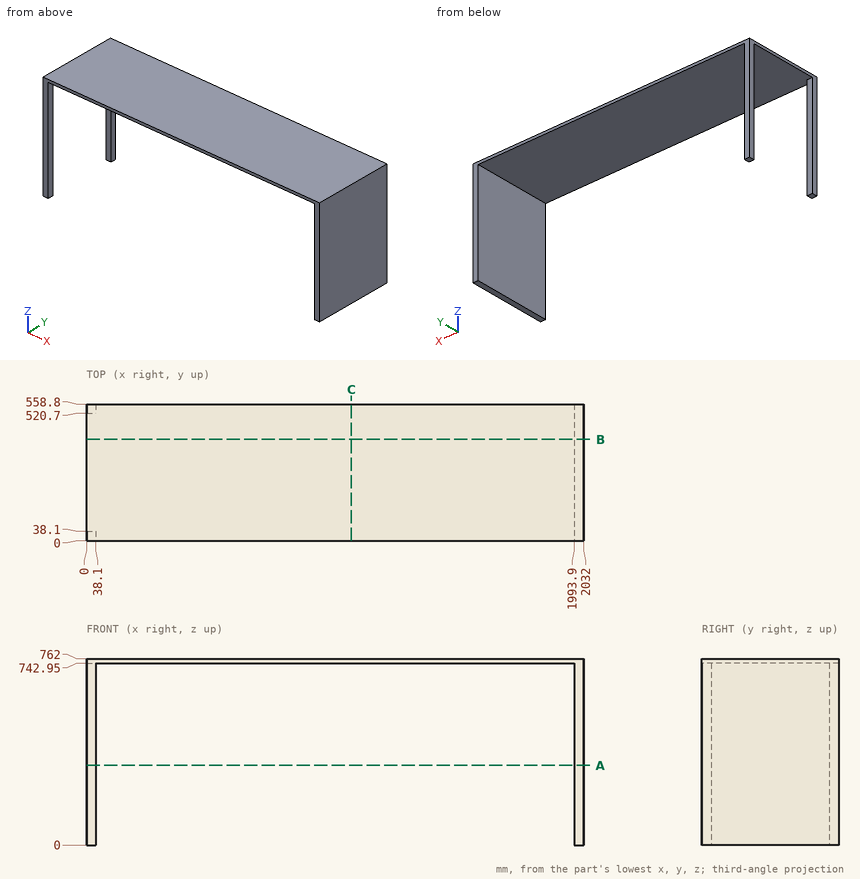
Could you check a few things on this drawing? It's one solid part, dimensions in mm from its lowest x, y, z. Give positions to 0.01 mm unless a question says otherwise; leave off trailing zeros. Write each loop counter-clockwise with the first axis right and the second up, starting at its lowest first coordinate (ties: lowest second). Pieces come first, ordered by that corner, then holes.
(1) Imagine slicing it at A-A, the plane z = 326.5. Write out the boundary of the cut face in (x, y), and give its area (3 significant figures).
Output values:
outline: (0, 0) - (38.1, 0) - (38.1, 38.1) - (0, 38.1) - close; (0, 520.7) - (38.1, 520.7) - (38.1, 558.8) - (0, 558.8) - close; (1993.9, 0) - (2032, 0) - (2032, 558.8) - (1993.9, 558.8) - close
area: 24,200 mm2
(2) If I drill on L1, parallel to X at y = 522.5, z = 251; L2, parallel to X at y = 406, z = 196.5; L3, parallel to Z at x = 1163, y = 388, over which ranges is the centre line in solid material (lowest first)?
Output values:
L1: x = 0 to 38.1, 1993.9 to 2032
L2: x = 1993.9 to 2032
L3: z = 742.95 to 762
(3) Imagine slicing it at C-C, the plane x = 1082. Write out the boundary of the cut face in (y, z), and give its area (3 significant figures).
Output values:
outline: (0, 742.95) - (558.8, 742.95) - (558.8, 762) - (0, 762) - close
area: 10,600 mm2
(4) Will these pins go through, and if not, where does the flat tip stop? pin 1 (5 mm diameter, centred on y = 248, z = 180.5, fed in from -X); pin 2 (19 mm diameter, centred on x = 11, z = 358.5, fed in from -Y).
Output values:
pin 1: stops at x = 1993.9
pin 2: stops at y = 0
(5) Imagine slicing it at B-B, the plane y = 414. Write out the boundary of the cut face in (x, z).
Output values:
outline: (0, 742.95) - (1993.9, 742.95) - (1993.9, 0) - (2032, 0) - (2032, 762) - (0, 762) - close
